from build123d import *

# Parameters (mm, degrees)
ESTRUSIONE_ESTRUSIONE1_DEPTH      = 78
ESTRUSIONE_ESTRUSIONE1_DEPTH_BACK = 78
SCHIZZO1_W                        = 169.9
SCHIZZO1_H                        = 163.8
SCHIZZO2_W                        = 169.9
SCHIZZO2_H                        = 163.8
SCHIZZO2_R                        = 40
TAGLIO_ESTRUSIONE1_DEPTH          = 50
SCHIZZO3_R                        = 35
TAGLIO_ESTRUSIONE2_DEPTH          = 10


with BuildPart() as part:
    # Schizzo1 → Estrusione-Estrusione1 (new, two sides: drawn at the far end of the back side and taken through both)
    with BuildSketch(Plane.XY.offset(-ESTRUSIONE_ESTRUSIONE1_DEPTH_BACK)):
        Rectangle(SCHIZZO1_W, SCHIZZO1_H)
    extrude(amount=ESTRUSIONE_ESTRUSIONE1_DEPTH + ESTRUSIONE_ESTRUSIONE1_DEPTH_BACK)

    # Schizzo2 → Taglio-Estrusione1 (cut)
    with BuildSketch(Plane.XY.offset(78)):
        Rectangle(SCHIZZO2_W, SCHIZZO2_H)
        Circle(SCHIZZO2_R, mode=Mode.SUBTRACT)
    extrude(amount=-TAGLIO_ESTRUSIONE1_DEPTH, mode=Mode.SUBTRACT)

    # Schizzo3 → Taglio-Estrusione2 (cut)
    with BuildSketch(Plane.XY.offset(78)):
        Circle(SCHIZZO3_R)
    extrude(amount=-TAGLIO_ESTRUSIONE2_DEPTH, mode=Mode.SUBTRACT)


solid = part.part
Could you check a few things on this model? Use its own coordinates, in mm. A direction names the side the tool comes from. Give positions to 0.01 mm unless a question says otherwise; leave off trailing zeros. Order: outer loops, then holes, each group sorted by start corner. A loop starts at its lowest first (then second) coordinate and runs counter-clockwise, first axis right, second up.
Item 1: If we mould it in two halves opening along X, with no side actions, what happens to faces 3 (the face through (-28, -21, 73)), 4 (the face through (84.95, -1, -26)), 5 (the face through (-84.95, -1, -26))? For each: pulls with the +X half, pulls with the -X half, needs draft (parallel to the pull), parting line crosses it, or undercut.
Item 2: I need wall thicknesses on line 1 (Y direction, x = 0, z = 71); line 2 (Z direction, x = -10, y = 43); line 3 (Z direction, x = -27.5, y = 21). Which ranges of each line are inside material? Lowest first, please.
Item 3: I'm going to push flat-ended pins straight in: pin 1 (5 mm diameter, centred on y = -21.5, z = 50, fed in from +X); pin 2 (1.5 mm diameter, centred on y = -5.5, z = 55, fed in from -X); pin 3 (10 mm diameter, centred on x = -9.5, z = 34.5, fed in from +Y). Where does each tip first touch, or does it pass through?
Item 4: If we section it at B-B, the plane x = 0: Write out the boundary of the cut face in (y, z).
Item 5: If we section it at C-C, the plane z = 37: Write out the boundary of the cut face in (x, y).
Item 6: If we section it at D-D, the plane x = -49.5: Write out the boundary of the cut face in (y, z), plus the area to 3 significant figures.
Item 7: If we section it at A-A, the plane y = 0: Write out the boundary of the cut face in (x, z).
Item 8: For faces 1 (the face through (-20, 38, 28)), 2 (the face through (-1, -81.9, -26)), which set-ups out of +Z, -Z, +X, -X, +Y, -Y let a thin tool reach every point of the face, with its end or its side?
Values:
1. face 3: undercut
1. face 4: pulls with the +X half
1. face 5: pulls with the -X half
2. line 1: y = -40 to -35, 35 to 40
2. line 2: z = -78 to 28
2. line 3: z = -78 to 68
3. pin 1: stops at x = 35.2
3. pin 2: stops at x = -39.72
3. pin 3: stops at y = 39.75
4. outline: (-81.9, -78) - (81.9, -78) - (81.9, 28) - (40, 28) - (40, 78) - (35, 78) - (35, 68) - (-35, 68) - (-35, 78) - (-40, 78) - (-40, 28) - (-81.9, 28) - close
5. outline: circle Ø80 at (0, 0)
6. outline: (-81.9, -78) - (81.9, -78) - (81.9, 28) - (-81.9, 28) - close
6. area: 17,400 mm2
7. outline: (-84.95, -78) - (84.95, -78) - (84.95, 28) - (40, 28) - (40, 78) - (35, 78) - (35, 68) - (-35, 68) - (-35, 78) - (-40, 78) - (-40, 28) - (-84.95, 28) - close
8. face 1: +Z
8. face 2: +Z, -Z, +X, -X, -Y
